Read the model definition and answer for the solid it produces. Units are mm, in the model's axes. A direction names the side the tool comes from. Round coordinates to 2 decimals unless told otherwise and drop trailing zeros. Write each loop counter-clockwise with the first axis right and the second up, starting at its lowest first coordinate (ties: lowest second). Pieces come first, ordered by that corner, then holes. Notation, with made-up numbers: (32, 2) -> (82, 2) arc R21 ccw to (82, 31) -> close; hole circle Ø4 at (55.5, 85.25). An arc over 180 degrees is marked (long way). Return JSON: item names as keys, results as strings.
from build123d import *

# Parameters (mm, degrees)
SKETCH1_W           = 145
SKETCH1_H           = 25
BOSS_EXTRUDE1_DEPTH = 10
SKETCH2_W           = 17.5
SKETCH2_H           = 32
BOSS_EXTRUDE2_DEPTH = 10
SKETCH4_W           = 73.5
SKETCH4_H           = 32
BOSS_EXTRUDE3_DEPTH = 10
CUT_EXTRUDE1_REACH  = 196.692
SKETCH5_R           = 2.25
SKETCH6_R           = 4.2
CUT_EXTRUDE2_DEPTH  = 2.4
CUT_EXTRUDE4_REACH  = 201.46
CUT_EXTRUDE4_START  = -5
SKETCH7_R           = 3.25
SKETCH8_R           = 2.25
CUT_EXTRUDE5_DEPTH  = 193.888568868
SKETCH9_W           = 7.3
SKETCH9_H           = 4
CUT_EXTRUDE6_DEPTH  = 10
CUT_EXTRUDE7_REACH  = 195.92
SKETCH10_R          = 4
SKETCH11_R          = 7
CUT_EXTRUDE8_DEPTH  = 2.5
CUT_EXTRUDE9_REACH  = 196.692
SKETCH12_R          = 1.75
CUT_EXTRUDE10_DEPTH = 3


with BuildPart() as part:
    # Sketch1 → Boss-Extrude1 (new body)
    with BuildSketch(Plane(origin=(0, 0, 0), x_dir=(1, 0, 0), z_dir=(0, 1, 0))):
        with Locations((72.5, 12.5)):
            Rectangle(SKETCH1_W, SKETCH1_H)
    extrude(amount=BOSS_EXTRUDE1_DEPTH)

    # Sketch2 → Boss-Extrude2 (add)
    with BuildSketch(Plane(origin=(0, 10, 0), x_dir=(1, 0, 0), z_dir=(0, 1, 0))):
        with Locations((153.75, 16)):
            Rectangle(SKETCH2_W, SKETCH2_H)
    extrude(amount=-BOSS_EXTRUDE2_DEPTH)

    # Sketch4 → Boss-Extrude3 (add)
    with BuildSketch(Plane.XZ):
        with Locations((154.25, -16)):
            Rectangle(SKETCH4_W, SKETCH4_H)
    extrude(amount=BOSS_EXTRUDE3_DEPTH)

    # Sketch5 → Cut-Extrude1 (cut, up to next)
    with BuildSketch(Plane.XZ.offset(10), mode=Mode.PRIVATE) as cut_extrude1_sk1:
        with Locations(Location((185, -7, 0), (0, 0, 270))):
            Circle(SKETCH5_R)
    cut_extrude1_tool1 = extrude(cut_extrude1_sk1.sketch, amount=-CUT_EXTRUDE1_REACH, mode=Mode.PRIVATE) & part.part
    # Sketch5 → Cut-Extrude1 (cut, up to next)
    with BuildSketch(Plane.XZ.offset(10), mode=Mode.PRIVATE) as cut_extrude1_sk2:
        with Locations(Location((152, -7, 0), (0, 0, 270))):
            Circle(SKETCH5_R)
    cut_extrude1_tool2 = extrude(cut_extrude1_sk2.sketch, amount=-CUT_EXTRUDE1_REACH, mode=Mode.PRIVATE) & part.part
    # Sketch5 → Cut-Extrude1 (cut, up to next)
    with BuildSketch(Plane.XZ.offset(10), mode=Mode.PRIVATE) as cut_extrude1_sk3:
        with Locations(Location((185, -25, 0), (0, 0, 270))):
            Circle(SKETCH5_R)
    cut_extrude1_tool3 = extrude(cut_extrude1_sk3.sketch, amount=-CUT_EXTRUDE1_REACH, mode=Mode.PRIVATE) & part.part
    # Sketch5 → Cut-Extrude1 (cut, up to next)
    with BuildSketch(Plane.XZ.offset(10), mode=Mode.PRIVATE) as cut_extrude1_sk4:
        with Locations(Location((152, -25, 0), (0, 0, 90))):
            Circle(SKETCH5_R)
    cut_extrude1_tool4 = extrude(cut_extrude1_sk4.sketch, amount=-CUT_EXTRUDE1_REACH, mode=Mode.PRIVATE) & part.part
    add(cut_extrude1_tool1.solids().sort_by_distance((185, -10, -7))[0], mode=Mode.SUBTRACT)
    add(cut_extrude1_tool2.solids().sort_by_distance((152, -10, -7))[0], mode=Mode.SUBTRACT)
    add(cut_extrude1_tool3.solids().sort_by_distance((185, -10, -25))[0], mode=Mode.SUBTRACT)
    add(cut_extrude1_tool4.solids().sort_by_distance((152, -10, -25))[0], mode=Mode.SUBTRACT)

    # Sketch6 → Cut-Extrude2 (cut)
    with BuildSketch(Plane.XZ.offset(10)):
        with Locations(Location((152, -7, 0), (0, 0, 270))):
            Circle(SKETCH6_R)
        with Locations(Location((185, -7, 0), (0, 0, 270))):
            Circle(SKETCH6_R)
        with Locations(Location((185, -25, 0), (0, 0, 90))):
            Circle(SKETCH6_R)
        with Locations(Location((152, -25, 0), (0, 0, 90))):
            Circle(SKETCH6_R)
    extrude(amount=-CUT_EXTRUDE2_DEPTH, mode=Mode.SUBTRACT)

    # Sketch7 → Cut-Extrude4 (cut, up to next)
    with BuildSketch(Plane.XZ.offset(7.6).offset(CUT_EXTRUDE4_START), mode=Mode.PRIVATE) as cut_extrude4_sk1:
        with Locations(Location((152, -7, 0), (0, 0, 270))):
            Circle(SKETCH7_R)
    cut_extrude4_tool1 = extrude(cut_extrude4_sk1.sketch, amount=-CUT_EXTRUDE4_REACH, mode=Mode.PRIVATE) & part.part
    # Sketch7 → Cut-Extrude4 (cut, up to next)
    with BuildSketch(Plane.XZ.offset(7.6).offset(CUT_EXTRUDE4_START), mode=Mode.PRIVATE) as cut_extrude4_sk2:
        with Locations(Location((185, -7, 0), (0, 0, 270))):
            Circle(SKETCH7_R)
    cut_extrude4_tool2 = extrude(cut_extrude4_sk2.sketch, amount=-CUT_EXTRUDE4_REACH, mode=Mode.PRIVATE) & part.part
    # Sketch7 → Cut-Extrude4 (cut, up to next)
    with BuildSketch(Plane.XZ.offset(7.6).offset(CUT_EXTRUDE4_START), mode=Mode.PRIVATE) as cut_extrude4_sk3:
        with Locations(Location((185, -25, 0), (0, 0, 270))):
            Circle(SKETCH7_R)
    cut_extrude4_tool3 = extrude(cut_extrude4_sk3.sketch, amount=-CUT_EXTRUDE4_REACH, mode=Mode.PRIVATE) & part.part
    # Sketch7 → Cut-Extrude4 (cut, up to next)
    with BuildSketch(Plane.XZ.offset(7.6).offset(CUT_EXTRUDE4_START), mode=Mode.PRIVATE) as cut_extrude4_sk4:
        with Locations(Location((152, -25, 0), (0, 0, 90))):
            Circle(SKETCH7_R)
    cut_extrude4_tool4 = extrude(cut_extrude4_sk4.sketch, amount=-CUT_EXTRUDE4_REACH, mode=Mode.PRIVATE) & part.part
    add(cut_extrude4_tool1.solids().sort_by_distance((152, -2.6, -7))[0], mode=Mode.SUBTRACT)
    add(cut_extrude4_tool2.solids().sort_by_distance((185, -2.6, -7))[0], mode=Mode.SUBTRACT)
    add(cut_extrude4_tool3.solids().sort_by_distance((185, -2.6, -25))[0], mode=Mode.SUBTRACT)
    add(cut_extrude4_tool4.solids().sort_by_distance((152, -2.6, -25))[0], mode=Mode.SUBTRACT)

    # Sketch8 → Cut-Extrude5 (cut, through all)
    with BuildSketch(Plane(origin=(0, 0, -25), x_dir=(-1, 0, 0), z_dir=(0, 0, -1))):
        with Locations((-137, 5)):
            Circle(SKETCH8_R)
        with Locations((-123, 5)):
            Circle(SKETCH8_R)
        with Locations(Location((-22, 5, 0), (0, 0, 180))):
            Circle(SKETCH8_R)
        with Locations(Location((-8, 5, 0), (0, 0, 180))):
            Circle(SKETCH8_R)
    extrude(amount=-CUT_EXTRUDE5_DEPTH, mode=Mode.SUBTRACT)

    # Sketch9 → Cut-Extrude6 (cut)
    with BuildSketch(Plane(origin=(0, 10, 0), x_dir=(1, 0, 0), z_dir=(0, 1, 0))):
        with Locations((137, 20)):
            Rectangle(SKETCH9_W, SKETCH9_H)
        with Locations((137, 5)):
            Rectangle(SKETCH9_W, SKETCH9_H)
        with Locations((123, 5)):
            Rectangle(SKETCH9_W, SKETCH9_H)
        with Locations((123, 20)):
            Rectangle(SKETCH9_W, SKETCH9_H)
        with Locations((8, 20)):
            Rectangle(SKETCH9_W, SKETCH9_H)
        with Locations((22, 20)):
            Rectangle(SKETCH9_W, SKETCH9_H)
        with Locations((22, 5)):
            Rectangle(SKETCH9_W, SKETCH9_H)
        with Locations((8, 5)):
            Rectangle(SKETCH9_W, SKETCH9_H)
    extrude(amount=-CUT_EXTRUDE6_DEPTH, mode=Mode.SUBTRACT)

    # Sketch10 → Cut-Extrude7 (cut, up to next)
    with BuildSketch(Plane(origin=(0, 0, 0), x_dir=(1, 0, 0), z_dir=(0, 1, 0)), mode=Mode.PRIVATE) as cut_extrude7_sk1:
        with Locations(Location((176, 16, 0), (0, 0, 270))):
            Circle(SKETCH10_R)
    cut_extrude7_tool1 = extrude(cut_extrude7_sk1.sketch, amount=-CUT_EXTRUDE7_REACH, mode=Mode.PRIVATE) & part.part
    add(cut_extrude7_tool1.solids().sort_by_distance((176, 0, -16))[0], mode=Mode.SUBTRACT)

    # Sketch11 → Cut-Extrude8 (cut)
    with BuildSketch(Plane.XZ.offset(10)):
        with Locations(Location((176, -16, 0), (0, 0, 270))):
            Circle(SKETCH11_R)
        with BuildLine():
            Line((160.5, -21.5), (160.5, -10.5))
            ThreePointArc((160.5, -10.5), (163.5, -7.5), (166.5, -10.5))
            Line((166.5, -10.5), (166.5, -21.5))
            ThreePointArc((166.5, -21.5), (163.5, -24.5), (160.5, -21.5))
        make_face()
    extrude(amount=-CUT_EXTRUDE8_DEPTH, mode=Mode.SUBTRACT)

    # Sketch12 → Cut-Extrude9 (cut, up to next)
    with BuildSketch(Plane(origin=(0, 10, 0), x_dir=(1, 0, 0), z_dir=(0, 1, 0)), mode=Mode.PRIVATE) as cut_extrude9_sk1:
        with Locations(Location((47.25, 12.5, 0), (0, 0, 270))):
            Circle(SKETCH12_R)
    cut_extrude9_tool1 = extrude(cut_extrude9_sk1.sketch, amount=-CUT_EXTRUDE9_REACH, mode=Mode.PRIVATE) & part.part
    # Sketch12 → Cut-Extrude9 (cut, up to next)
    with BuildSketch(Plane(origin=(0, 10, 0), x_dir=(1, 0, 0), z_dir=(0, 1, 0)), mode=Mode.PRIVATE) as cut_extrude9_sk2:
        with Locations(Location((72.5, 12.5, 0), (0, 0, 270))):
            Circle(SKETCH12_R)
    cut_extrude9_tool2 = extrude(cut_extrude9_sk2.sketch, amount=-CUT_EXTRUDE9_REACH, mode=Mode.PRIVATE) & part.part
    # Sketch12 → Cut-Extrude9 (cut, up to next)
    with BuildSketch(Plane(origin=(0, 10, 0), x_dir=(1, 0, 0), z_dir=(0, 1, 0)), mode=Mode.PRIVATE) as cut_extrude9_sk3:
        with Locations(Location((97.75, 12.5, 0), (0, 0, 270))):
            Circle(SKETCH12_R)
    cut_extrude9_tool3 = extrude(cut_extrude9_sk3.sketch, amount=-CUT_EXTRUDE9_REACH, mode=Mode.PRIVATE) & part.part
    add(cut_extrude9_tool1.solids().sort_by_distance((47.25, 10, -12.5))[0], mode=Mode.SUBTRACT)
    add(cut_extrude9_tool2.solids().sort_by_distance((72.5, 10, -12.5))[0], mode=Mode.SUBTRACT)
    add(cut_extrude9_tool3.solids().sort_by_distance((97.75, 10, -12.5))[0], mode=Mode.SUBTRACT)

    # Sketch13 → Cut-Extrude10 (cut)
    with BuildSketch(Plane(origin=(0, 10, 0), x_dir=(1, 0, 0), z_dir=(0, 1, 0))):
        Polygon((75.964101615, 12.5), (74.232050808, 15.5), (70.767949192, 15.5), (69.035898385, 12.5), (70.767949192, 9.5), (74.232050808, 9.5), align=None)
        Polygon((50.714101615, 12.5), (48.982050808, 15.5), (45.517949192, 15.5), (43.785898385, 12.5), (45.517949192, 9.5), (48.982050808, 9.5), align=None)
        Polygon((101.214101615, 12.5), (99.482050808, 15.5), (96.017949192, 15.5), (94.285898385, 12.5), (96.017949192, 9.5), (99.482050808, 9.5), align=None)
    extrude(amount=-CUT_EXTRUDE10_DEPTH, mode=Mode.SUBTRACT)


solid = part.part
Item 1: Section A-A (x = 97.75) is taken. Give the vertices of the cut face in (y, z).
Worked answers:
{"outline": "(0, -25) -> (10, -25) -> (10, -15.5) -> (7, -15.5) -> (7, -14.25) -> (0, -14.25) -> close; (0, -10.75) -> (7, -10.75) -> (7, -9.5) -> (10, -9.5) -> (10, 0) -> (0, 0) -> close"}
Item 2: For a pull along X with two mould halves and no side action, classify faces 4 (the flat face through (154, -2, -32)), 5 (the flat face through (117.5, -5, -16)), 6 (the flat face through (47, 9, -9.5)), 7 (the cylindrical face through (5.752, 4.901, -23.521)) as released by +X, released by -X, zero draft, split by the parting line, or undercut.
Worked answers:
{"face 4": "zero draft", "face 5": "released by -X", "face 6": "undercut", "face 7": "undercut"}
Item 3: Straight lines are drawn through the part: L1, parallel to Z at x = 119.5, y = 4.5; L2, parallel to X at y = 8.5, z = -18.5; L3, parallel to Z at x = 152, y = 4.25. For each, find the intervals that lie inside material, in ascending order. Write a range as [from, to].
Worked answers:
{"L1": "z = [-25, -22], [-18, -7], [-3, 0]", "L2": "x = [0, 4.35], [11.65, 18.35], [25.65, 119.35], [126.65, 133.35], [140.65, 162.5]", "L3": "z = [-32, -28.25], [-21.75, -10.25], [-3.75, 0]"}
Item 4: Section D-D (y = 5) is taken. State how many separate pieces and enclosed holes the cut face has, then the cut area to 3 significant figures.
Worked answers:
{"separate pieces": "5", "enclosed holes": "5", "area": "3,550 mm2"}
Item 5: Flat-ended cylindrical pins translate along their axes: pin 1 (12 mm diameter, centred on x = 102, y = 2, fed in from -Z); pin 2 (4 mm diameter, centred on x = 151.5, z = -26, fed in from -Y); pin 3 (3 mm diameter, centred on x = 170.5, z = -20, fed in from +Y). Find the tip coordinate at first contact, or state that the pin passes through.
Worked answers:
{"pin 1": "stops at z = -25", "pin 2": "stops at y = -7.6", "pin 3": "stops at y = 0"}
Item 6: Section B-B (y = -5) is taken. Give the vertices of the cut face in (x, z).
Worked answers:
{"outline": "(117.5, -32) -> (191, -32) -> (191, 0) -> (117.5, 0) -> close; hole circle Ø4.5 at (152, -25); hole circle Ø4.5 at (152, -7); hole circle Ø8 at (176, -16); hole circle Ø4.5 at (185, -25); hole circle Ø4.5 at (185, -7)"}
Item 7: A tool of negligible diameter and unlimited length cuts with its end or side. For faces 1 (the flat face through (131, 0, -28)), 2 (the flat face through (4.35, 5, -20)), 3 (the flat face through (119.35, 5, -5)), from which of +Z, -Z, +X, -X, +Y, -Y can it reach the whole face along a straight path? Write none if from no direction.
Worked answers:
{"face 1": "-Z, -X, +Y", "face 2": "+Y, -Y", "face 3": "+Y"}
Item 8: Section C-C (x = 123) is taken. Give the vertices of the cut face in (y, z).
Worked answers:
{"outline": "(-10, -32) -> (0, -32) -> (0, -25) -> (2.75, -25) -> (2.75, -22) -> (0, -22) -> (0, -18) -> (2.75, -18) -> (2.75, -7) -> (0, -7) -> (0, -3) -> (2.75, -3) -> (2.75, 0) -> (-10, 0) -> close; (7.25, -25) -> (10, -25) -> (10, -22) -> (7.25, -22) -> close; (7.25, -18) -> (10, -18) -> (10, -7) -> (7.25, -7) -> close; (7.25, -3) -> (10, -3) -> (10, 0) -> (7.25, 0) -> close"}
